from build123d import *

# Parameters (mm, degrees)
PAD_DEPTH    = 42.5
SKETCH001_W  = 150
SKETCH001_H  = 50
POCKET_DEPTH = 39


with BuildPart() as part:
    # Sketch → Pad (new body, symmetric)
    with BuildSketch(Plane.YZ):
        Polygon((105, 30), (135, 10), (135, 0), (0, 0), (0, 30), align=None)
    extrude(amount=PAD_DEPTH, both=True)

    # Sketch001 → Pocket (cut, symmetric)
    with BuildSketch(Plane.YZ):
        with Locations((78, 28)):
            Rectangle(SKETCH001_W, SKETCH001_H)
    extrude(amount=POCKET_DEPTH, both=True, mode=Mode.SUBTRACT)


solid = part.part
Could you check a few things on this model? Use its own coordinates, in mm. A direction names the side the tool comes from. Coordinates: 2 decimals unless noted, no trailing zeros. Order: outer loops, then holes, each group sorted by start corner. A loop starts at its lowest first (then second) coordinate and runs counter-clockwise, first axis right, second up.
Q1. Which directions (+Z, -Z, +X, -X, +Y, -Y) give clear straight access to the entire face, cutting with the end or side of a thin tool? Please do faces 1 (the flat face through (39, 68, 17)), 2 (the flat face through (1, 0, 15)).
Q2. Suppose I cut it at B-B on y = 75.5. Please give me the cut outline in (x, z).
Q3. Suppose I cut it at A-A on z = 15. Please give me the cut outline in (x, y), and give its area (3 significant figures).
Q4. Please list where these lines run through material, in increasing order: L1, parallel to X at y = 74, z = 3.5; L2, parallel to Z at x = -36, y = 52.
Q5. Will these pins go through, and if not, where does the flat tip stop? pin 1 (23.5 mm diameter, centred on x = 2.5, y = 84.5, fed in from +Z); pin 2 (12 mm diameter, centred on x = -30.5, z = 20, fed in from +Y).
Q6. Suppose I cut it at C-C on x = 10. Please give me the cut outline in (y, z), and give its area (3 significant figures).
Q7. Thinking about a two-plate mould opening in X: for faces 3 (the flat face through (1, 68, 3)), 4 (the flat face through (-42.5, 68, 15)), 5 (the flat face through (42.5, 68, 15)), 6 (the flat face through (-41, 120, 20)), which applies, released by +X, released by -X, zero draft, split by the parting line, or undercut?
Answer:
1. face 1: +Z, +Y
1. face 2: +Z, -Z, +X, -X, -Y
2. outline: (-42.5, 0) - (42.5, 0) - (42.5, 30) - (39, 30) - (39, 3) - (-39, 3) - (-39, 30) - (-42.5, 30) - close
3. outline: (-42.5, 0) - (42.5, 0) - (42.5, 127.5) - (39, 127.5) - (39, 3) - (-39, 3) - (-39, 127.5) - (-42.5, 127.5) - close
3. area: 1,130 mm2
4. L1: x = -42.5 to -39, 39 to 42.5
4. L2: z = 0 to 3
5. pin 1: stops at z = 3
5. pin 2: stops at y = 3
6. outline: (0, 0) - (135, 0) - (135, 3) - (3, 3) - (3, 30) - (0, 30) - close
6. area: 486 mm2
7. face 3: undercut
7. face 4: released by -X
7. face 5: released by +X
7. face 6: zero draft
